For this review, take the finished solid that the model builds, in its own axes (mm). A direction names the side the tool comes from. Round coordinates to 2 decimals unless told otherwise and drop trailing zeros. Order: outer loops, then holes, each group sorted by start corner. A loop starts at its lowest first (then second) coordinate and runs counter-clockwise, first axis right, second up. Notation, with made-up numbers: M -4,-23.75 L 32,-23.75 A18 ccw 32,-2.75 Z; hole C -33,44 d4. An arc over 180 degrees is marked long. Put each result on its own line as item: value.
from build123d import *

# Parameters (mm, degrees)
F1_DEPTH  = 32
F2_R      = 6
F3_DEPTH  = 10
F4_R      = 3.4
F5_DEPTH  = 22.001
F7_DEPTH  = 32.001
F9_DEPTH  = 11
F11_DEPTH = 25
F12_R     = 3
F13_R     = 3


# Not quite as in the source:
# - the arcs of a loft's sections are written as splines that run evenly, so that the points pair up as in the source's solid


with BuildPart() as f1:
    # F0 (on Front) → F1 (new body)
    with BuildSketch(Plane.XZ):
        Polygon((-16, 17), (-16, -17), (16, -17), (16, 17), (7.4519659326, 17), (10.15, 13), (-10.15, 13), (-7.4519659326, 17), align=None)
    extrude(amount=F1_DEPTH)

    # F2 (on face) → F3 (cut)
    with BuildSketch(Plane(origin=(-16, 0, 0), x_dir=(0, -1, 0), z_dir=(-1, 0, 0))):
        with Locations((16, 5)):
            Circle(F2_R)
    extrude(amount=-F3_DEPTH, mode=Mode.SUBTRACT)

    # F4 (on face) → F5 (cut, through all)
    with BuildSketch(Plane(origin=(-6, 0, 0), x_dir=(0, -1, 0), z_dir=(-1, 0, 0))):
        with Locations((16, 5)):
            Circle(F4_R)
    extrude(amount=-F5_DEPTH, mode=Mode.SUBTRACT)

    # F6 (on face) → F7 (cut, through all)
    with BuildSketch(Plane.XZ.offset(32)):
        with BuildLine():
            Line((0.75, 13), (-0.75, 13))
            Line((-0.75, 13), (-0.75, -10.5))
            Line((-0.75, -10.5), (-8.0952624903, -10.5))
            ThreePointArc((-8.0952624903, -10.5), (-14, -11.25), (-8.0952624903, -12))
            Line((-8.0952624903, -12), (0.75, -12))
            Line((0.75, -12), (0.75, 13))
        make_face()
    extrude(amount=-F7_DEPTH, mode=Mode.SUBTRACT)

    # F8 (on face) → F9 (cut)
    with BuildSketch(Plane.YZ.offset(16)):
        Polygon((-12.9689110868, -0.25), (-9.9378221735, 5), (-12.9689110868, 10.25), (-19.0310889132, 10.25), (-22.0621778265, 5), (-19.0310889132, -0.25), align=None)
    extrude(amount=-F9_DEPTH, mode=Mode.SUBTRACT)

    # F10 (on face) → F11 (join)
    with BuildSketch(Plane(origin=(0, 0, -17), x_dir=(1, 0, 0), z_dir=(0, 0, -1))):
        with BuildLine():
            ThreePointArc((11.234, 15.4002133713), (11.85, 16), (11.234, 16.5997866287))
            ThreePointArc((11.234, 16.5997866287), (7.9549512883, 23.9549512883), (0.5997866287, 27.234))
            ThreePointArc((0.5997866287, 27.234), (0, 27.85), (-0.5997866287, 27.234))
            ThreePointArc((-0.5997866287, 27.234), (-7.9549512883, 23.9549512883), (-11.234, 16.5997866287))
            ThreePointArc((-11.234, 16.5997866287), (-11.85, 16), (-11.234, 15.4002133713))
            ThreePointArc((-11.234, 15.4002133713), (-7.9549512883, 8.0450487117), (-0.5997866287, 4.766))
            ThreePointArc((-0.5997866287, 4.766), (0, 4.15), (0.5997866287, 4.766))
            ThreePointArc((0.5997866287, 4.766), (7.9549512883, 8.0450487117), (11.234, 15.4002133713))
        make_face()
    extrude(amount=F11_DEPTH)

    # F12
    f12_edges = [f1.edges().sort_by_distance(p)[0] for p in [
        (-16, -16, -17),
    ]]
    fillet(f12_edges, radius=F12_R)

    # F13
    f13_edges = [f1.edges().sort_by_distance(p)[0] for p in [
        (16, -16, -17),
    ]]
    fillet(f13_edges, radius=F13_R)

    # F11_face (on face) → F16 section 0
    with BuildSketch(Plane(origin=(0, -16, -42), x_dir=(1, 0, 0), z_dir=(0, 0, -1))):
        with BuildLine():
            add(Edge.make_bspline(
                [(0.5997866287, -11.234), (1.9704441734, -11.1608201827), (3.3271537618, -10.8340484232), (5.834489174, -9.7162386482), (6.984369661, -8.9255329157), (8.9255329157, -6.984369661), (9.7162386482, -5.834489174), (10.8340484232, -3.3271537618), (11.1608201827, -1.9704441734), (11.234, -0.5997866287)],
                knots=[0, 0, 0, 0, 0.25, 0.25, 0.5, 0.5, 0.75, 0.75, 1, 1, 1, 1], degree=3))
            add(Edge.make_bspline(
                [(11.234, -0.5997866287), (11.3049732474, -0.6016799219), (11.376267359, -0.5908445992), (11.5106795168, -0.5450568557), (11.5737621993, -0.5101164815), (11.6838785828, -0.4204642218), (11.7308833124, -0.3657759235), (11.8029722112, -0.2434389451), (11.8280374139, -0.1758224517), (11.853109213, -0.0360563953), (11.853109213, 0.0360563953), (11.8280374139, 0.1758224517), (11.8029722112, 0.2434389451), (11.7308833124, 0.3657759235), (11.6838785828, 0.4204642218), (11.5737621993, 0.5101164815), (11.5106795168, 0.5450568557), (11.376267359, 0.5908445992), (11.3049732474, 0.6016799219), (11.234, 0.5997866287)],
                knots=[0, 0, 0, 0, 0.1111111111, 0.1111111111, 0.2222222222, 0.2222222222, 0.3333333333, 0.3333333333, 0.4444444444, 0.4444444444, 0.5555555556, 0.5555555556, 0.6666666667, 0.6666666667, 0.7777777778, 0.7777777778, 0.8888888889, 0.8888888889, 1, 1, 1, 1], degree=3))
            add(Edge.make_bspline(
                [(11.234, 0.5997866287), (11.1608201827, 1.9704441734), (10.8340484232, 3.3271537618), (9.7162386482, 5.834489174), (8.9255329157, 6.984369661), (6.984369661, 8.9255329157), (5.834489174, 9.7162386482), (3.3271537618, 10.8340484232), (1.9704441734, 11.1608201827), (0.5997866287, 11.234)],
                knots=[0, 0, 0, 0, 0.25, 0.25, 0.5, 0.5, 0.75, 0.75, 1, 1, 1, 1], degree=3))
            add(Edge.make_bspline(
                [(0.5997866287, 11.234), (0.6016799219, 11.3049732474), (0.5908445992, 11.376267359), (0.5450568557, 11.5106795168), (0.5101164815, 11.5737621993), (0.4204642218, 11.6838785828), (0.3657759235, 11.7308833124), (0.2434389451, 11.8029722112), (0.1758224517, 11.8280374139), (0.0360563953, 11.853109213), (-0.0360563953, 11.853109213), (-0.1758224517, 11.8280374139), (-0.2434389451, 11.8029722112), (-0.3657759235, 11.7308833124), (-0.4204642218, 11.6838785828), (-0.5101164815, 11.5737621993), (-0.5450568557, 11.5106795168), (-0.5908445992, 11.376267359), (-0.6016799219, 11.3049732474), (-0.5997866287, 11.234)],
                knots=[0, 0, 0, 0, 0.1111111111, 0.1111111111, 0.2222222222, 0.2222222222, 0.3333333333, 0.3333333333, 0.4444444444, 0.4444444444, 0.5555555556, 0.5555555556, 0.6666666667, 0.6666666667, 0.7777777778, 0.7777777778, 0.8888888889, 0.8888888889, 1, 1, 1, 1], degree=3))
            add(Edge.make_bspline(
                [(-0.5997866287, 11.234), (-1.9704441734, 11.1608201827), (-3.3271537618, 10.8340484232), (-5.834489174, 9.7162386482), (-6.984369661, 8.9255329157), (-8.9255329157, 6.984369661), (-9.7162386482, 5.834489174), (-10.8340484232, 3.3271537618), (-11.1608201827, 1.9704441734), (-11.234, 0.5997866287)],
                knots=[0, 0, 0, 0, 0.25, 0.25, 0.5, 0.5, 0.75, 0.75, 1, 1, 1, 1], degree=3))
            add(Edge.make_bspline(
                [(-11.234, 0.5997866287), (-11.3049732474, 0.6016799219), (-11.376267359, 0.5908445992), (-11.5106795168, 0.5450568557), (-11.5737621993, 0.5101164815), (-11.6838785828, 0.4204642218), (-11.7308833124, 0.3657759235), (-11.8029722112, 0.2434389451), (-11.8280374139, 0.1758224517), (-11.853109213, 0.0360563953), (-11.853109213, -0.0360563953), (-11.8280374139, -0.1758224517), (-11.8029722112, -0.2434389451), (-11.7308833124, -0.3657759235), (-11.6838785828, -0.4204642218), (-11.5737621993, -0.5101164815), (-11.5106795168, -0.5450568557), (-11.376267359, -0.5908445992), (-11.3049732474, -0.6016799219), (-11.234, -0.5997866287)],
                knots=[0, 0, 0, 0, 0.1111111111, 0.1111111111, 0.2222222222, 0.2222222222, 0.3333333333, 0.3333333333, 0.4444444444, 0.4444444444, 0.5555555556, 0.5555555556, 0.6666666667, 0.6666666667, 0.7777777778, 0.7777777778, 0.8888888889, 0.8888888889, 1, 1, 1, 1], degree=3))
            add(Edge.make_bspline(
                [(-11.234, -0.5997866287), (-11.1608201827, -1.9704441734), (-10.8340484232, -3.3271537618), (-9.7162386482, -5.834489174), (-8.9255329157, -6.984369661), (-6.984369661, -8.9255329157), (-5.834489174, -9.7162386482), (-3.3271537618, -10.8340484232), (-1.9704441734, -11.1608201827), (-0.5997866287, -11.234)],
                knots=[0, 0, 0, 0, 0.25, 0.25, 0.5, 0.5, 0.75, 0.75, 1, 1, 1, 1], degree=3))
            add(Edge.make_bspline(
                [(-0.5997866287, -11.234), (-0.6016799219, -11.3049732474), (-0.5908445992, -11.376267359), (-0.5450568557, -11.5106795168), (-0.5101164815, -11.5737621993), (-0.4204642218, -11.6838785828), (-0.3657759235, -11.7308833124), (-0.2434389451, -11.8029722112), (-0.1758224517, -11.8280374139), (-0.0360563953, -11.853109213), (0.0360563953, -11.853109213), (0.1758224517, -11.8280374139), (0.2434389451, -11.8029722112), (0.3657759235, -11.7308833124), (0.4204642218, -11.6838785828), (0.5101164815, -11.5737621993), (0.5450568557, -11.5106795168), (0.5908445992, -11.376267359), (0.6016799219, -11.3049732474), (0.5997866287, -11.234)],
                knots=[0, 0, 0, 0, 0.1111111111, 0.1111111111, 0.2222222222, 0.2222222222, 0.3333333333, 0.3333333333, 0.4444444444, 0.4444444444, 0.5555555556, 0.5555555556, 0.6666666667, 0.6666666667, 0.7777777778, 0.7777777778, 0.8888888889, 0.8888888889, 1, 1, 1, 1], degree=3))
        make_face()
    # F15 (on offset) → F16 section 1
    with BuildSketch(Plane(origin=(0, 0, -43.5), x_dir=(1, 0, 0), z_dir=(0, 0, -1))):
        with BuildLine():
            add(Edge.make_bspline(
                [(0.5464722617, 5.7645777778), (1.8862858976, 5.8361108296), (3.2113491637, 6.1740163798), (5.6322529271, 7.3316411864), (6.7271409022, 8.1509049669), (7.6239507036, 9.1488777804)],
                knots=[0, 0, 0, 0, 0.5, 0.5, 1, 1, 1, 1], degree=3))
            add(Edge.make_bspline(
                [(7.6239507036, 9.1488777804), (8.5207605051, 10.1468505938), (9.2187864201, 11.3227471207), (10.112059537, 13.8531489393), (10.306955274, 15.2066586259), (10.2354222222, 16.5464722617)],
                knots=[0, 0, 0, 0, 0.5, 0.5, 1, 1, 1, 1], degree=3))
            add(Edge.make_bspline(
                [(10.2354222222, 16.5464722617), (10.1638891704, 17.8862858976), (9.8259836202, 19.2113491637), (8.6683588136, 21.6322529271), (7.8490950331, 22.7271409022), (6.8511222196, 23.6239507036)],
                knots=[0, 0, 0, 0, 0.5, 0.5, 1, 1, 1, 1], degree=3))
            add(Edge.make_bspline(
                [(6.8511222196, 23.6239507036), (5.8531494062, 24.5207605051), (4.6772528793, 25.2187864201), (2.1468510607, 26.112059537), (0.7933413741, 26.306955274), (-0.5464722617, 26.2354222222)],
                knots=[0, 0, 0, 0, 0.5, 0.5, 1, 1, 1, 1], degree=3))
            add(Edge.make_bspline(
                [(-0.5464722617, 26.2354222222), (-1.8862858976, 26.1638891704), (-3.2113491637, 25.8259836202), (-5.6322529271, 24.6683588136), (-6.7271409022, 23.8490950331), (-7.6239507036, 22.8511222196)],
                knots=[0, 0, 0, 0, 0.5, 0.5, 1, 1, 1, 1], degree=3))
            add(Edge.make_bspline(
                [(-7.6239507036, 22.8511222196), (-8.5207605051, 21.8531494062), (-9.2187864201, 20.6772528793), (-10.112059537, 18.1468510607), (-10.306955274, 16.7933413741), (-10.2354222222, 15.4535277383)],
                knots=[0, 0, 0, 0, 0.5, 0.5, 1, 1, 1, 1], degree=3))
            add(Edge.make_bspline(
                [(-10.2354222222, 15.4535277383), (-10.1638891704, 14.1137141024), (-9.8259836202, 12.7886508363), (-8.6683588136, 10.3677470729), (-7.8490950331, 9.2728590978), (-6.8511222196, 8.3760492964)],
                knots=[0, 0, 0, 0, 0.5, 0.5, 1, 1, 1, 1], degree=3))
            add(Edge.make_bspline(
                [(-6.8511222196, 8.3760492964), (-5.8531494062, 7.4792394949), (-4.6772528793, 6.7812135799), (-2.1468510607, 5.887940463), (-0.7933413741, 5.693044726), (0.5464722617, 5.7645777778)],
                knots=[0, 0, 0, 0, 0.5, 0.5, 1, 1, 1, 1], degree=3))
        make_face()
    loft(ruled=True)


solid = f1.part
(1) Add section C-C on x = 14.5. Give the boundary of the cut face in (y, z).
A:
outline: M -32,-16.6 L 0,-16.6 L 0,17 L -32,17 Z; hole M -22.06,5 L -19.03,-0.25 L -12.97,-0.25 L -9.94,5 L -12.97,10.25 L -19.03,10.25 Z
(2) To check wall thickness, follow L1, parallel to X at y = -6.5, z = -11.25; L2, parallel to Z at x = 6.5, y = -17; L3, parallel to X at y = -17, z = 11. State the ranges of each line that lie inside material, in increasing order.
A:
L1: x = -16 to -14, 0.75 to 16
L2: z = -43.5 to -0.25, 10.25 to 13
L3: x = -16 to -0.75, 0.75 to 16
(3) Draft analysis for pull direction X (two halves, no side actions). For faces 5 (the face through (10.577, -11.475, 2.338)), 6 (the face through (0.01, -27.85, -29.32)), 7 (the face through (-4, -16, -12)), state which applies: released by +X, released by -X, zero draft, split by the parting line, or undercut.
A:
face 5: zero draft
face 6: split by the parting line
face 7: undercut
(4) For faces 1 (the face through (11, -16, -0.25)), 2 (the face through (0.75, -16, 0)), 3 (the face through (-8.8, -15.8, 15)), 4 (the face through (16, -16, -2)), list the 3-axis set-ups (+Z, -Z, +X, -X, +Y, -Y) from which the entire face can be reached by the end or side of a thin tool; tool diameter is ignored.
A:
face 1: +X
face 2: +Z, +Y, -Y
face 3: +Y, -Y
face 4: +Z, -Z, +X, +Y, -Y
(5) Insertion check: pin 1 Ø3 at (x, y) = (-2.5, -5) entering from +Z; pin 2 Ø7 at (y, z) = (-16, 5) entering from -X; pin 3 Ø8 at (y, z) = (-16, 5) entering from +X; pin 4 Ø6.5 at (x, y) = (12, -16) entering from -Z. Each pin has a flat end and moves straight along its axis. Give the tip position at first contact, or say it passes through.
A:
pin 1: stops at z = 13
pin 2: stops at x = -6
pin 3: stops at x = 5
pin 4: stops at z = -43.5
(6) Add section A-A on z = -25. Give the boundary of the cut face in (x, y).
A:
outline: M -11.23,-16.6 A11.25 ccw -0.6,-27.23 A0.6 ccw long 0.6,-27.23 A11.25 ccw 11.23,-16.6 A0.6 ccw long 11.23,-15.4 A11.25 ccw 0.6,-4.77 A0.6 ccw long -0.6,-4.77 A11.25 ccw -11.23,-15.4 A0.6 ccw long Z
(7) Add section B-B on y = -3. Give the boundary of the cut face in (x, z).
A:
outline: M -16,-14 A3 ccw -13,-17 L 13,-17 A3 ccw 16,-14 L 16,17 L 7.45,17 L 10.15,13 L 0.75,13 L 0.75,-12 L -8.1,-12 A3 cw long -8.1,-10.5 L -0.75,-10.5 L -0.75,13 L -10.15,13 L -7.45,17 L -16,17 Z
